```python
from build123d import *

# Parameters (mm, degrees)
SKETCH1_W           = 80
SKETCH1_H           = 100
BOSS_EXTRUDE1_DEPTH = 2
CHAMFER1_SIZE       = 2
CHAMFER2_SIZE       = 6
BOSS_EXTRUDE2_DEPTH = 6.5
CHAMFER3_SIZE       = 1
CHAMFER4_SIZE       = 1
FILLET1_R           = 2


with BuildPart() as part:
    # Sketch1 → Boss-Extrude1 (new body)
    with BuildSketch(Plane(origin=(0, 0, 0), x_dir=(1, 0, 0), z_dir=(0, 1, 0))):
        Rectangle(SKETCH1_W, SKETCH1_H)
    extrude(amount=BOSS_EXTRUDE1_DEPTH)

    # Chamfer1
    chamfer1_edges = [part.edges().sort_by_distance(p)[0] for p in [
        (-40, 1, 50),
    ]]
    chamfer(chamfer1_edges, length=CHAMFER1_SIZE)

    # Chamfer2
    chamfer2_edges = [part.edges().sort_by_distance(p)[0] for p in [
        (40, 1, -50),
    ]]
    chamfer(chamfer2_edges, length=CHAMFER2_SIZE)

    # Sketch3 → Boss-Extrude2 (add)
    with BuildSketch(Plane.XZ):
        Polygon((26, 46), (36, 36), (36, -36), (26, -46), (-26, -46), (-36, -36), (-36, 36), (-26, 46), align=None)
        Polygon((25.171572875, 44), (34, 35.171572875), (34, -35.171572875), (25.171572875, -44), (-25.171572875, -44), (-34, -35.171572875), (-34, 35.171572875), (-25.171572875, 44), align=None, mode=Mode.SUBTRACT)
    extrude(amount=BOSS_EXTRUDE2_DEPTH)

    # Chamfer3
    chamfer3_edges = [part.edges().sort_by_distance(p)[0] for p in [
        (0, -6.5, 46),
        (-31, -6.5, 41),
        (-36, -6.5, 0),
        (-31, -6.5, -41),
        (0, -6.5, -46),
        (31, -6.5, -41),
        (36, -6.5, 0),
        (31, -6.5, 41),
    ]]
    chamfer(chamfer3_edges, length=CHAMFER3_SIZE)

    # Chamfer4
    chamfer4_edges = [part.edges().sort_by_distance(p)[0] for p in [
        (0, 0, 46),
        (-31, 0, 41),
        (-36, 0, 0),
        (-31, 0, -41),
        (0, 0, -46),
        (31, 0, -41),
        (36, 0, 0),
        (31, 0, 41),
    ]]
    chamfer(chamfer4_edges, length=CHAMFER4_SIZE)

    # Fillet1
    fillet1_edges = [part.edges().sort_by_distance(p)[0] for p in [
        (0, 0, 44),
        (-29.585786438, 0, 39.585786438),
        (-34, 0, 0),
        (-29.585786438, 0, -39.585786438),
        (0, 0, -44),
        (29.585786438, 0, -39.585786438),
        (34, 0, 0),
        (29.585786438, 0, 39.585786438),
    ]]
    fillet(fillet1_edges, radius=FILLET1_R)


solid = part.part
```
The listing builds one solid part. Answer for the finished solid, in the listing's coordinates (mm). A direction names the side the tool comes from. Give positions to 0.01 mm unless a question says otherwise; leave off trailing zeros. Order: outer loops, then holes, each group sorted by start corner. A loop starts at its lowest first (then second) coordinate and runs counter-clockwise, first axis right, second up. Notation, with made-up numbers: (-27.5, 40.5) -> (-7.5, 40.5) arc R35 ccw to (-7.5, 72.5) -> close; hole circle Ø11 at (-36, -37.75). An arc over 180 degrees is marked (long way). Write each question's results on one line, items separated by ' | '.
Q1. Which of the six approach directions +Z, -Z, +X, -X, +Y, -Y give full straight-line access (tool end or side, diameter ignored) to faces 5 (the face through (-0.35, -0.6, -43.43)), 6 (the face through (0, -3, -46)), 7 (the face through (-31, -3, 41)), 8 (the face through (0, -3, 46)), 9 (the face through (31, -3, 41))?
Checked values:
face 5: -Y | face 6: -Z, +X, -X, -Y | face 7: +Z, -X, -Y | face 8: +Z, +X, -X, -Y | face 9: +Z, +X, -Y
Q2. The part is cut by section A-A, the plane z = -17. Give the vertices of the cut face in (x, y).
Checked values:
outline: (-40, 0) -> (-37, 0) -> (-36, -1) -> (-36, -5.5) -> (-35, -6.5) -> (-34, -6.5) -> (-34, -2) arc R2 cw to (-32, 0) -> (32, 0) arc R2 cw to (34, -2) -> (34, -6.5) -> (35, -6.5) -> (36, -5.5) -> (36, -1) -> (37, 0) -> (40, 0) -> (40, 2) -> (-40, 2) -> close
Q3. Straight lines are drawn through the part: probe 1 along Z at (x, y) = (-22.5, -3.75); probe 2 along X at (y, z) = (-2.75, 29.5); probe 3 along Y at (x, z) = (26, 20.5). For each, find the intervals that lie inside material, in ascending order. Write a range as from..to.
Checked values:
probe 1: z = -46..-44, 44..46 | probe 2: x = -36..-34, 34..36 | probe 3: y = 0..2
Q4. Each of these flat-tipped pins is pushed along its axis until it touches: P1, Ø1.3, axis at x = -7.5, y = -2.5, coming from the +Z side; P2, Ø3.5, axis at y = -5, z = 10, coming from the -X side; P3, Ø3.5, axis at y = -3.5, z = -4, coming from the +X side. Where does it stop, or does it pass through?
Checked values:
P1: stops at z = 46 | P2: stops at x = -36 | P3: stops at x = 36
Q5. Determine the mould class of faces 1 (the face through (-30.57, -6.01, -40.71)), 2 (the face through (31, -3, -41)), 3 (the face through (29.52, -4.22, 39.65)), 4 (the face through (-39, 0, 3)) for opening direction X: pulls with the +X half, pulls with the -X half, needs draft (parallel to the pull), parting line crosses it, or undercut.
Checked values:
face 1: pulls with the -X half | face 2: pulls with the +X half | face 3: undercut | face 4: needs draft
Q6. The part is cut by section B-B, the plane x = 1.5. Give the vertices of the cut face in (y, z).
Checked values:
outline: (-6.5, -45) -> (-5.5, -46) -> (-1, -46) -> (0, -47) -> (0, -50) -> (2, -50) -> (2, 50) -> (0, 50) -> (0, 47) -> (-1, 46) -> (-5.5, 46) -> (-6.5, 45) -> (-6.5, 44) -> (-2, 44) arc R2 cw to (0, 42) -> (0, -42) arc R2 cw to (-2, -44) -> (-6.5, -44) -> close
